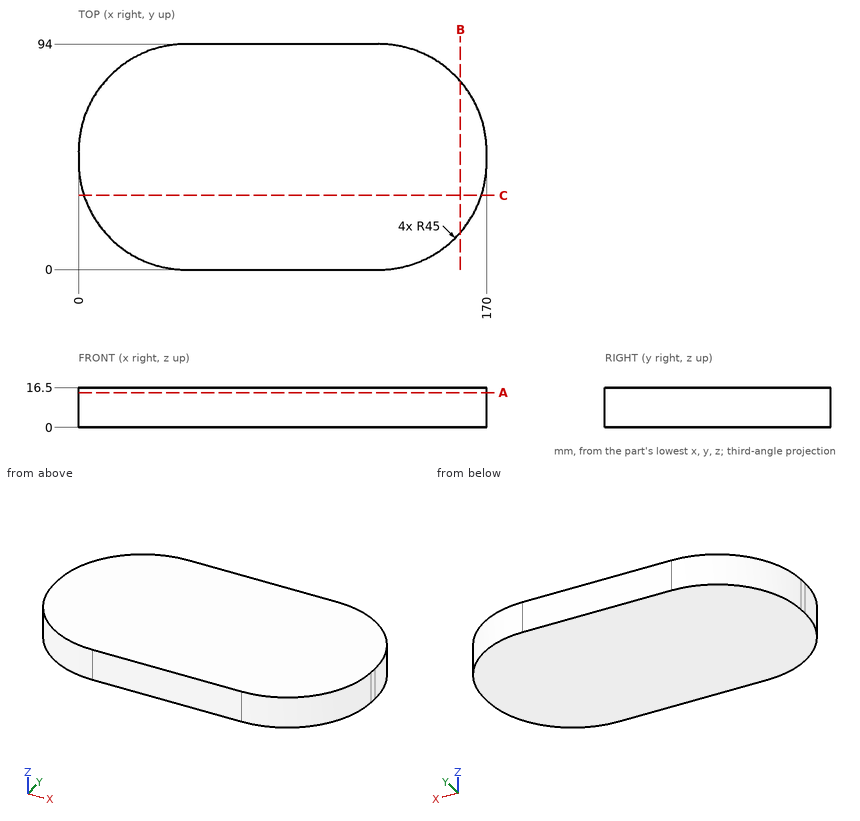
Part print with two shaded views. Sizes in mm from the minimum x, y, z corner. Round coordinates to 2 decimals unless told otherwise and drop trailing zeros. Order: outer loops, then holes, each group sorted by start corner. A loop starts at its lowest first (then second) coordinate and runs counter-clockwise, first axis right, second up. Notation, with made-up numbers: (3.25, 32) - (56.25, 32) arc R13 ccw to (56.25, 52) - close; hole circle Ø3 at (12.5, 78.5). An arc over 180 degrees is marked (long way). Answer as CSV lines item,"result". Start each with the question number.
1. Saw through at A-A, the plane z = 14.5. Write the cut outline in (x, y).
2. Saw through at C-C, the plane y = 31. Write the cut outline in (x, z).
3. Saw through at B-B, the plane x = 159. Write the cut outline in (y, z), and give its area (3 significant figures).
4. Pin check, flat tips, straight feed: pin 1 (2 mm diameter, centred on x = 136.5, z = 6, fed in from -Y); pin 2 (4 mm diameter, centred on y = 24, z = 4, fed in from +X). Stop position of each tip, or through.
5. Drill centre lines: L1, parallel to Y at x = 15, z = 11; L2, parallel to X at y = 61.5, z = 5.25; L3, parallel to X at y = 19.5, z = 6. Where is each one in solid material? Low to high. Write a range as [from, to].
Model answer:
1,outline,"(0, 45) arc R45 ccw to (45, 0) - (125, 0) arc R45 ccw to (170, 45) - (170, 49) arc R45 ccw to (125, 94) - (45, 94) arc R45 ccw to (0, 49) - close"
2,outline,"(2.23, 0) - (167.77, 0) - (167.77, 16.5) - (2.23, 16.5) - close"
3,outline,"(15.52, 0) - (78.48, 0) - (78.48, 16.5) - (15.52, 16.5) - close"
3,area,"1,040 mm²"
4,pin 1,"stops at y = 1.24"
4,pin 2,"stops at x = 165.79"
5,L1,"y = [11.46, 82.54]"
5,L2,"x = [1.77, 168.23]"
5,L3,"x = [7.92, 162.08]"
